Build history of the part. All positions in model axes, mm. A direction names the side the tool comes from. Give positions to 0.01 mm unless a question says otherwise; leave off trailing zeros. Loops run counter-clockwise (first coordinate to the right, second up) from the corner with the lowest first, then second, coordinate; pieces in that order, holes last. Notation, with made-up numbers: M 27.5,58 L 64.5,58 A33 cw 64.5,86 Z; hole C -25.75,57.25 d2. An arc over 180 degrees is marked long. Put each result on its own line as item: value.
```python
from build123d import *

# Parameters (mm, degrees)
EXTRUDE_1_DEPTH      = 20
SKETCH_3_R           = 2
EXTRUDE_2_DEPTH      = 15
EXTRUDE_2_DEPTH_BACK = 35
SKETCH_4_R           = 2
CUT_EXTRUDE_1_DEPTH  = 2


with BuildPart() as part:
    # 草图1 → 凸台-拉伸1 (new body)
    with BuildSketch(Plane.XY):
        Polygon((-38.9636651, 28.845358616), (-38.9636651, -11.154641384), (-36.9636651, -11.154641384), (-36.9636651, 28.845358616), (-6.9636651, 28.845358616), (-6.9636651, -11.154641384), (-4.9636651, -11.154641384), (-4.9636651, 30.845358616), (-38.9636651, 30.845358616), align=None)
    extrude(amount=EXTRUDE_1_DEPTH)

    # 草图3 → 凸台-拉伸2 (add, two sides)
    with BuildSketch(Plane.ZY.offset(38.9636651)) as extrude_2_sk:
        with Locations((10, -1.154641384)):
            Circle(SKETCH_3_R)
    extrude(amount=EXTRUDE_2_DEPTH)
    extrude(extrude_2_sk.sketch, amount=-EXTRUDE_2_DEPTH_BACK)

    # 草图4 → 切除-拉伸1 (cut)
    with BuildSketch(Plane(origin=(0, 30.845358616, 0), x_dir=(1, 0, 0), z_dir=(0, 1, 0))):
        with Locations((-12.9636651, -10)):
            Circle(SKETCH_4_R)
    extrude(amount=-CUT_EXTRUDE_1_DEPTH, mode=Mode.SUBTRACT)


solid = part.part
```
Q1. Slice it at C-C (x = -31). List the corners of the cut face in (y, z), and give its area (3 significant figures).
Here are the results:
outline: C -1.15,10 d4; M 28.85,0 L 30.85,0 L 30.85,20 L 28.85,20 Z
area: 52.6 mm²
Q2. Tool access for faces 5 (the cylindrical face through (-46.36, -2.37, 8.41)), 6 (the flat face through (-53.964, -1, 10)), 7 (the cylindrical face through (-4.47, -2.37, 8.41)): list every direction of +Z, -Z, +X, -X, +Y, -Y with a clear straight run to the whole face (end or side of a thin tool).
Here are the results:
face 5: -X
face 6: +Z, -Z, -X, +Y, -Y
face 7: +X
Q3. Probe line 1 (X direction, y = 12, z = 13.25); line 2 (X direction, y = 29.7, z = 10); line 3 (Y direction, x = -25.5, z = 4.5). List the from-to ranges inside material, lowest first. Write a range as from..to.
Here are the results:
line 1: -38.96..-36.96, -6.96..-4.96
line 2: -38.96..-14.96, -10.96..-4.96
line 3: 28.85..30.85
Q4. Slice it at B-B (z = 14.75). List the corners of the cut face in (x, y), and give its area (3 significant figures).
Here are the results:
outline: M -38.96,-11.15 L -36.96,-11.15 L -36.96,28.85 L -6.96,28.85 L -6.96,-11.15 L -4.96,-11.15 L -4.96,30.85 L -38.96,30.85 Z
area: 228 mm²
Q5. Drop flat-ended pins along their axis: pin 1 Ø3 at (x, y) = (-44, 1) entering from -Z; pin 2 Ø1 at (y, z) = (21.5, 17) entering from -X; pin 3 Ø12 at (y, z) = (19, 11) entering from +X. Give the stop position or say it passes through.
Here are the results:
pin 1: z = 8.11
pin 2: x = -38.96
pin 3: x = -4.96
Q6. Slice it at A-A (y = 21.5). List the corners of the cut face in (x, z).
Here are the results:
outline: M -38.96,0 L -36.96,0 L -36.96,20 L -38.96,20 Z; M -6.96,0 L -4.96,0 L -4.96,20 L -6.96,20 Z
Q7. Slice it at D-D (z = 10). List the corners of the cut face in (x, y).
Here are the results:
outline: M -53.96,-3.15 L -38.96,-3.15 L -38.96,-11.15 L -36.96,-11.15 L -36.96,-3.15 L -6.96,-3.15 L -6.96,-11.15 L -4.96,-11.15 L -4.96,-3.15 L -3.96,-3.15 L -3.96,0.85 L -4.96,0.85 L -4.96,30.85 L -10.96,30.85 L -10.96,28.85 L -6.96,28.85 L -6.96,0.85 L -36.96,0.85 L -36.96,28.85 L -14.96,28.85 L -14.96,30.85 L -38.96,30.85 L -38.96,0.85 L -53.96,0.85 Z
Q8. Mould opens along Y. For faces 1 (the flat face through (-6, -11.155, 10)), 2 (the cylindrical face through (-22.17, -2.37, 8.41)), 3 (the cylindrical face through (-11.888, 29.859, 8.314)), 4 (the flat face through (-22, 30.845, 10)) say: pulls with the +Y half, pulls with the -Y half, needs draft (parallel to the pull), parting line crosses it, or undercut.
Here are the results:
face 1: pulls with the -Y half
face 2: undercut
face 3: needs draft
face 4: pulls with the +Y half
